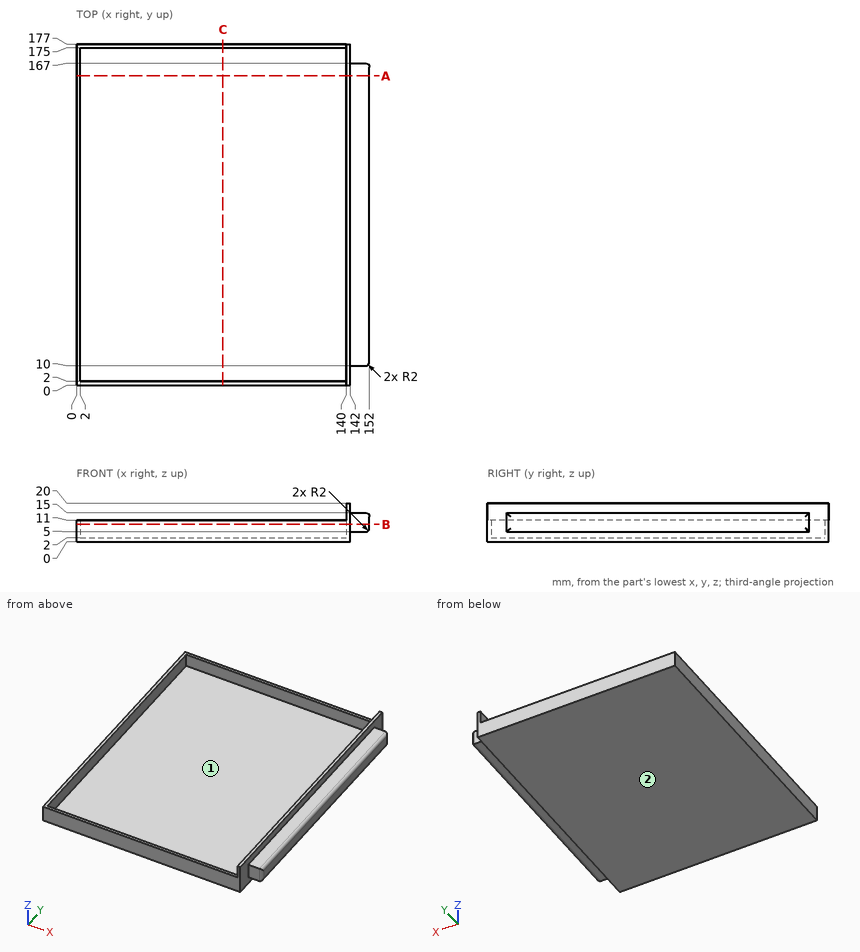
Source: three-view drawing plus pictorial views. Frame: mm from the lowest corner of the part. Round coordinates to 2 decimals unless told otherwise and drop trailing zeros. Loops run counter-clockwise (first coordinate to the right, second up) from the corner with the lowest first, then second, coordinate; pieces in that order, holes last. Notation, with made-up numbers: (60, 26) - (103, 26) arc R19 cw to (103, 54) - close; hole circle Ø8 at (10.25, 5). An arc over 180 degrees is marked (long way). Write item = value, one per line. Start each with the question number.
Item 1: Material intervals for line 1 (Y direction, x = 100.5, z = 5); line 2 (X direction, y = 150, z = 7.5); line 3 (X direction, y = 11.5, z = 3.25), sorted ascending.
Item 2: First-contact query: pin 1 Ø10 at (x, z) = (80, 16.5) entering from -Y; pin 2 Ø4 at (x, z) = (146, 10) entering from +Y; pin 3 Ø6 at (x, y) = (135, 101) entering from +Z; pin 4 Ø9 at (x, y) = (148, 54.5) entering from -Z. Flat tips, straight axial feed; report the tip coordinate or a pass-through.
Item 3: Mould query, pull axis X, two halves, no side actions, for the marked faces 1 and 2. Classes: released by +X, released by -X, zero draft, split by the parting line, or undercut.
Item 4: Section query C-C on x = 76. Output: boundary loops of the cut face in (y, z).
Item 5: Section query B-B on z = 9. Output: boundary loops of the cut face in (x, y).
Item 6: Section query A-A on y = 160.5. Output: boundary loops of the cut face in (x, z), plus the area to 3 significant figures.
Results list:
q1.line_1 = 0 to 2, 175 to 177
q1.line_2 = 0 to 2, 140 to 152
q1.line_3 = 0 to 2, 140 to 142
q2.pin_1 = through
q2.pin_2 = 167
q2.pin_3 = 2
q2.pin_4 = 5
q3.face_1 = undercut
q3.face_2 = zero draft
q4.outline = (0, 0) - (177, 0) - (177, 11) - (175, 11) - (175, 2) - (2, 2) - (2, 11) - (0, 11) - close
q5.outline = (0, 0) - (142, 0) - (142, 10) - (150, 10) arc R2 ccw to (152, 12) - (152, 165) arc R2 ccw to (150, 167) - (142, 167) - (142, 177) - (0, 177) - close; hole (2, 2) - (140, 2) - (140, 175) - (2, 175) - close
q6.outline = (0, 0) - (142, 0) - (142, 5) - (150, 5) arc R2 ccw to (152, 7) - (152, 13) arc R2 ccw to (150, 15) - (142, 15) - (142, 20) - (140, 20) - (140, 2) - (2, 2) - (2, 11) - (0, 11) - close
q6.area = 436 mm²
